from build123d import *

# Parameters (mm, degrees)
F0_R     = 10
F1_DEPTH = 20
F2_R     = 4.25
F3_DEPTH = 20.001
F4_W     = 23.145964
F4_H     = 10
F5_DEPTH = 2


with BuildPart() as f1:
    # F0 (on Top) → F1 (new body)
    with BuildSketch(Plane.XY):
        Circle(F0_R)
    extrude(amount=-F1_DEPTH)

    # F2 (on Top) → F3 (cut, through all)
    with BuildSketch(Plane.XY):
        Circle(F2_R)
    extrude(amount=-F3_DEPTH, mode=Mode.SUBTRACT)

    # F4 (on face) → F5 (cut)
    with BuildSketch(Plane.XY):
        Rectangle(F4_W, F4_H)
    extrude(amount=-F5_DEPTH, mode=Mode.SUBTRACT)


solid = f1.part
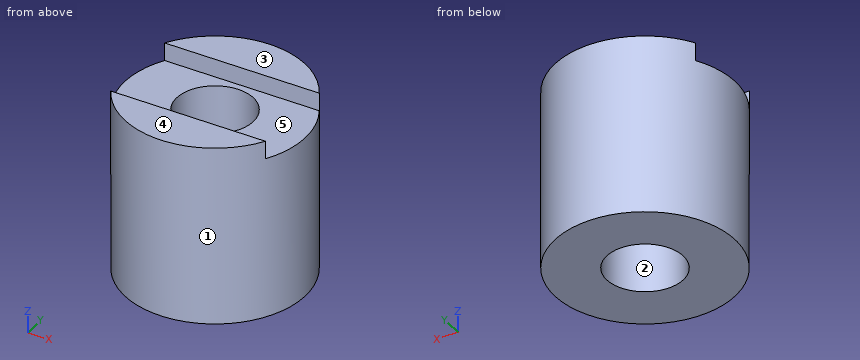
Can you work these out from the model? Positions are in its coordinate system, mm. Face numbers are marked on the shaded views. A direction names the side the tool comes from. Round coordinates to 2 decimals unless told otherwise and drop trailing zeros. Write each loop counter-clockwise with the first axis right and the second up, starting at its lowest first coordinate (ties: lowest second). Pieces come first, ordered by that corner, then holes. Notation, with made-up numbers: (79.25, -30) -> (111.25, -30) arc R25 ccw to (111.25, -16) -> close; hole circle Ø8 at (38.25, -3.75). An arc over 180 degrees is marked (long way). One line per question, with ' | ' between items. Start each with the question number.
1) Suppose I cut it at C-C on z = -10.5. Write out the boundary of the cut face in (x, y), then the cut area to 3 significant figures.
2) If we mould it in two halves opening along X, with no side actions, what happens to the marked faces 1, 2 and 3? For each: released by +X, released by -X, zero draft, split by the parting line, or undercut.
3) Suppose I cut it at A-A on y = 0. Write out the boundary of the cut face in (x, z).
4) Suppose I cut it at D-D on x = 3.75. Write out the boundary of the cut face in (y, z).
5) On a 3-axis mill with a long thin cutter (end or side, diameter ignored), from which of +Z, -Z, +X, -X, +Y, -Y can I reach the whole of each face in a straight line? I mean the marked faces 4 and 5. Say none if no direction works.
6) I need wall thicknesses on line 1 (Y direction, x = 0, z = -15.25); line 2 (Y direction, x = 3.5, z = -13.25); line 3 (X direction, y = -0.5, z = -14). Which ranges of each line are inside material? Lowest first, please. Write a range as [from, to].
7) I'm going to push flat-ended pins straight in: P1, Ø4, axis at x = 2, y = 2.5, coming from the +Z side; P2, Ø3, axis at y = -5.5, z = -8.5, coming from the -X side; P3, Ø0.6, axis at x = -2, z = -1, coming from the +Y side. Where does each tip first touch, or does it pass through?
8) Suppose I cut it at B-B on x = 0. Write out the boundary of the cut face in (y, z).
Return value:
1) outline: circle Ø20 at (0, 0); hole circle Ø8.5 at (0, 0) | area: 257 mm2
2) face 1: split by the parting line | face 2: undercut | face 3: zero draft
3) outline: (-10, -20) -> (-4.25, -20) -> (-4.25, -2) -> (-10, -2) -> close; (4.25, -20) -> (10, -20) -> (10, -2) -> (4.25, -2) -> close
4) outline: (-9.27, -20) -> (-2, -20) -> (-2, -2) -> (-5, -2) -> (-5, 0) -> (-9.27, 0) -> close; (2, -20) -> (9.27, -20) -> (9.27, 0) -> (5, 0) -> (5, -2) -> (2, -2) -> close
5) face 4: +Z, +X, -X, +Y, -Y | face 5: +Z, +X, -X
6) line 1: y = [-10, -4.25], [4.25, 10] | line 2: y = [-9.37, -2.41], [2.41, 9.37] | line 3: x = [-9.99, -4.22], [4.22, 9.99]
7) P1: stops at z = -2 | P2: stops at x = -9.17 | P3: stops at y = 9.85
8) outline: (-10, -20) -> (-4.25, -20) -> (-4.25, -2) -> (-5, -2) -> (-5, 0) -> (-10, 0) -> close; (4.25, -20) -> (10, -20) -> (10, 0) -> (5, 0) -> (5, -2) -> (4.25, -2) -> close
